For this review, take the finished solid that the model builds, in its own axes (mm). Face numbers are marked on the shaded views. A direction names the side the tool comes from. Round coordinates to 2 decimals unless told otherwise and drop trailing zeros. Order: outer loops, then holes, each group sorted by start corner. A loop starts at its lowest first (then second) coordinate and runs counter-clockwise, first axis right, second up. Notation, with made-up numbers: (54.5, 16.25) -> (97.5, 16.25) arc R18 cw to (97.5, 39.25) -> close; hole circle Ø5 at (-24, 35). An arc over 180 degrees is marked (long way). Use a Markdown table: item, result. Add a question column.
1) Clearance check with flat-ended pins moving along their axes: P1, Ø0.6, axis at x = -73, z = 15.5, coming from the -Y side; P2, Ø16, axis at y = -0.5, z = 84, coming from the +X side; P3, Ø22, axis at y = 9, z = 87.5, coming from the -X side. State where each tip first meets the part, or that it passes through.
2) Consider section C-C (y = -6). State the section outline as (x, z) points, plus the area to 3 significant figures.
3) Consider section A-A (z = 7). Give the number of separate pieces and of enclosed holes in the cut face, plus the area to 3 significant figures.
4) Machinability: for the marked faces 1, 2 and 3, which of the approach directions +Z, -Z, +X, -X, +Y, -Y give a long, thin tool a straight path to every point of the face, cutting with its end or side? Answer none if there is none.
5) Consider section D-D (z = 73.5). State the section outline as (x, y) points.
6) Wall thickness on line 1 along X through (y, z) = (12, 91.5); line 2 along Y through (x, z) = (40.5, 76.2); line 3 along Z through (x, y) = (-33, 0): over which ranges is each line inside the solid? List them lowest first. Write a range as [from, to].
7) Consider section B-B (x = 34.5). State the section outline as (y, z) points, plus the area to 3 significant figures.
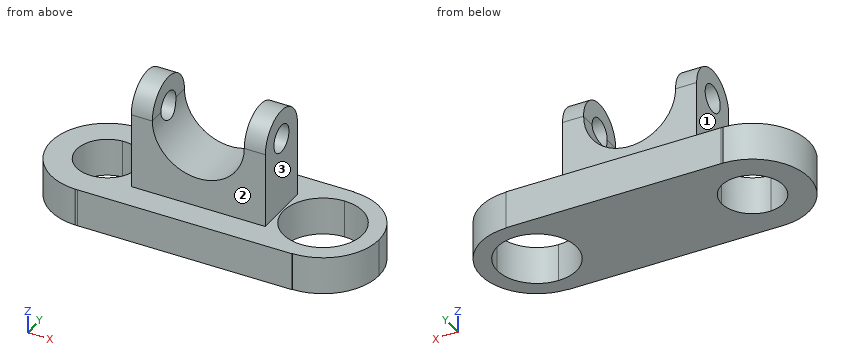
```python
from build123d import *

# Parameters (mm, degrees)
F1_DEPTH  = 76.2
F2_DEPTH  = 25.4
F3_R      = 31.0113659553
F4_DEPTH  = 48.768
F5_W      = 14.2128238031
F5_H      = 19.8651105165
F7_W      = 14.2128238031
F7_H      = 19.8651105165
F9_R      = 9.3175662763
F10_DEPTH = 120.904


with BuildPart() as f1:
    # F0 (on Top) → F1 (new body)
    with BuildSketch(Plane.XY):
        with BuildLine():
            ThreePointArc((-39.4395748653, 19.8651105165), (-35.2913919529, 10.3150682913), (-33.8736140697, 0))
            ThreePointArc((-33.8736140697, 0), (-35.2913919529, -10.3150682913), (-39.4395748653, -19.8651105165))
            Line((-39.4395748653, -19.8651105165), (41.0163370235, -19.8651105165))
            ThreePointArc((41.0163370235, -19.8651105165), (35.3919404434, 0), (41.0163370235, 19.8651105165))
            Line((41.0163370235, 19.8651105165), (-39.4395748653, 19.8651105165))
        make_face()
        with BuildLine():
            ThreePointArc((-39.4395748653, -19.8651105165), (-35.2913919529, -10.3150682913), (-33.8736140697, 0))
            ThreePointArc((-33.8736140697, 0), (-35.2913919529, 10.3150682913), (-39.4395748653, 19.8651105165))
            Line((-39.4395748653, 19.8651105165), (-45.2241897583, 19.8651105165))
            Line((-45.2241897583, 19.8651105165), (-45.2241897583, -19.8651105165))
            Line((-45.2241897583, -19.8651105165), (-39.4395748653, -19.8651105165))
        make_face()
        with BuildLine():
            Line((45.2241897583, 19.8651105165), (41.0163370235, 19.8651105165))
            ThreePointArc((41.0163370235, 19.8651105165), (35.3919404434, 0), (41.0163370235, -19.8651105165))
            Line((41.0163370235, -19.8651105165), (45.2241897583, -19.8651105165))
            Line((45.2241897583, -19.8651105165), (45.2241897583, 19.8651105165))
        make_face()
    extrude(amount=F1_DEPTH)

    # F0 (on Top) → F2 (join)
    with BuildSketch(Plane.XY):
        with BuildLine():
            Line((-45.2241897583, 19.8651105165), (-39.4395748653, 19.8651105165))
            ThreePointArc((-39.4395748653, 19.8651105165), (-53.1034448807, 33.1757028633), (-71.4977306772, 38.2277779281))
            Line((-71.4977306772, 38.2277779281), (-72.7147387814, 38.2277779281))
            ThreePointArc((-72.7147387814, 38.2277779281), (-73.0001282654, 38.2221694419), (-73.2854679227, 38.2144304102))
            Line((-73.2854679227, 38.2144304102), (-73.2854679227, 20.8573796838))
            ThreePointArc((-73.2854679227, 20.8573796838), (-57.7572646523, 15.1831464436), (-51.2155459374, 0))
            ThreePointArc((-51.2155459374, 0), (-57.7572646523, -15.1831464436), (-73.2854679227, -20.8573796838))
            Line((-73.2854679227, -20.8573796838), (-73.2854679227, -38.2144304102))
            ThreePointArc((-73.2854679227, -38.2144304102), (-73.0001282654, -38.2221694419), (-72.7147387814, -38.2277779281))
            Line((-72.7147387814, -38.2277779281), (-71.4977306772, -38.2277779281))
            ThreePointArc((-71.4977306772, -38.2277779281), (-53.1034448807, -33.1757028633), (-39.4395748653, -19.8651105165))
            Line((-39.4395748653, -19.8651105165), (-45.2241897583, -19.8651105165))
            Line((-45.2241897583, -19.8651105165), (-45.2241897583, 19.8651105165))
        make_face()
        with BuildLine():
            ThreePointArc((-71.4977306772, 38.2277779281), (-53.1034448807, 33.1757028633), (-39.4395748653, 19.8651105165))
            Line((-39.4395748653, 19.8651105165), (41.0163370235, 19.8651105165))
            ThreePointArc((41.0163370235, 19.8651105165), (54.80358066, 33.0807990839), (73.2854679227, 37.8935274793))
            Line((73.2854679227, 37.8935274793), (73.2854679227, 38.2277779281))
            Line((73.2854679227, 38.2277779281), (-71.4977306772, 38.2277779281))
        make_face()
        with BuildLine():
            Line((41.0163370235, -19.8651105165), (-39.4395748653, -19.8651105165))
            ThreePointArc((-39.4395748653, -19.8651105165), (-53.1034448807, -33.1757028633), (-71.4977306772, -38.2277779281))
            Line((-71.4977306772, -38.2277779281), (73.2854679227, -38.2277779281))
            Line((73.2854679227, -38.2277779281), (73.2854679227, -37.8935274793))
            ThreePointArc((73.2854679227, -37.8935274793), (54.80358066, -33.0807990839), (41.0163370235, -19.8651105165))
        make_face()
        with BuildLine():
            Line((-72.7147387814, 38.2277779281), (-71.4977306772, 38.2277779281))
            ThreePointArc((-71.4977306772, 38.2277779281), (-72.1062347293, 38.2326206596), (-72.7147387814, 38.2277779281))
        make_face()
        with BuildLine():
            ThreePointArc((73.2854679227, 37.8935274793), (54.80358066, 33.0807990839), (41.0163370235, 19.8651105165))
            Line((41.0163370235, 19.8651105165), (45.2241897583, 19.8651105165))
            Line((45.2241897583, 19.8651105165), (45.2241897583, -19.8651105165))
            Line((45.2241897583, -19.8651105165), (41.0163370235, -19.8651105165))
            ThreePointArc((41.0163370235, -19.8651105165), (54.80358066, -33.0807990839), (73.2854679227, -37.8935274793))
            Line((73.2854679227, -37.8935274793), (73.2854679227, -26.8271780999))
            ThreePointArc((73.2854679227, -26.8271780999), (46.4582898228, 0), (73.2854679227, 26.8271780999))
            Line((73.2854679227, 26.8271780999), (73.2854679227, 37.8935274793))
        make_face()
        with BuildLine():
            ThreePointArc((-72.7147387814, -38.2277779281), (-72.1062347293, -38.2326206596), (-71.4977306772, -38.2277779281))
            Line((-71.4977306772, -38.2277779281), (-72.7147387814, -38.2277779281))
        make_face()
        with BuildLine():
            ThreePointArc((-73.2854679227, 38.2144304102), (-73.0001282654, 38.2221694419), (-72.7147387814, 38.2277779281))
            Line((-72.7147387814, 38.2277779281), (-73.2854679227, 38.2277779281))
            Line((-73.2854679227, 38.2277779281), (-73.2854679227, 38.2144304102))
        make_face()
        with BuildLine():
            ThreePointArc((111.178995402, 0), (100.0802381664, 26.7947702437), (73.2854679227, 37.8935274793))
            Line((73.2854679227, 37.8935274793), (73.2854679227, 26.8271780999))
            ThreePointArc((73.2854679227, 26.8271780999), (92.2551474772, 18.9696795545), (100.1126460226, 0))
            ThreePointArc((100.1126460226, 0), (92.2551474772, -18.9696795545), (73.2854679227, -26.8271780999))
            Line((73.2854679227, -26.8271780999), (73.2854679227, -37.8935274793))
            ThreePointArc((73.2854679227, -37.8935274793), (100.0802381664, -26.7947702437), (111.178995402, 0))
        make_face()
        with BuildLine():
            Line((-73.2854679227, -38.2277779281), (-72.7147387814, -38.2277779281))
            ThreePointArc((-72.7147387814, -38.2277779281), (-73.0001282654, -38.2221694419), (-73.2854679227, -38.2144304102))
            Line((-73.2854679227, -38.2144304102), (-73.2854679227, -38.2277779281))
        make_face()
        with BuildLine():
            Line((-73.2854679227, 20.8573796838), (-73.2854679227, 38.2144304102))
            ThreePointArc((-73.2854679227, 38.2144304102), (-110.3388553889, 0), (-73.2854679227, -38.2144304102))
            Line((-73.2854679227, -38.2144304102), (-73.2854679227, -20.8573796838))
            ThreePointArc((-73.2854679227, -20.8573796838), (-92.9969235211, 0), (-73.2854679227, 20.8573796838))
        make_face()
    extrude(amount=F2_DEPTH)

    # F3 (on face) → F4 (cut)
    with BuildSketch(Plane.XZ.offset(19.8651105165)):
        with Locations((0, 76.2)):
            Circle(F3_R)
    extrude(amount=-F4_DEPTH, mode=Mode.SUBTRACT)

    # F5 (on face) → F6 (revolve)
    with BuildSketch(Plane.XY.offset(76.2)):
        with Locations((-38.1177778568, 9.9325552583)):
            Rectangle(F5_W, F5_H)
    revolve(axis=Axis((-38.1177778568, 0, 76.2), (1, 0, 0)))

    # F7 (on face) → F8 (revolve)
    with BuildSketch(Plane.XY.offset(76.2)):
        with Locations((38.1177778568, 9.9325552583)):
            Rectangle(F7_W, F7_H)
    revolve(axis=Axis((38.1177778568, 0, 76.2), (1, 0, 0)))

    # F9 (on face) → F10 (cut)
    with BuildSketch(Plane.YZ.offset(45.2241897583)):
        with Locations((0, 76.2)):
            Circle(F9_R)
    extrude(amount=-F10_DEPTH, mode=Mode.SUBTRACT)


solid = f1.part
```
Results list:
| question | item | result |
|---|---|---|
| 1 | P1 | y = -38.23 |
| 1 | P2 | x = 45.22 |
| 1 | P3 | x = -45.22 |
| 2 | outline | (-109.87, 0) -> (-92.12, 0) -> (-92.12, 25.4) -> (-109.87, 25.4) -> close; (-52.1, 0) -> (47.14, 0) -> (47.14, 25.4) -> (45.22, 25.4) -> (45.22, 69.07) -> (30.18, 69.07) arc R31.01 cw to (-30.18, 69.07) -> (-45.22, 69.07) -> (-45.22, 25.4) -> (-52.1, 25.4) -> close; (-45.22, 83.33) -> (-31.01, 83.33) -> (-31.01, 95.14) -> (-45.22, 95.14) -> close; (31.01, 83.33) -> (45.22, 83.33) -> (45.22, 95.14) -> (31.01, 95.14) -> close; (99.43, 0) -> (110.7, 0) -> (110.7, 25.4) -> (99.43, 25.4) -> close |
| 2 | area | 6,470 mm2 |
| 3 | separate pieces | 1 |
| 3 | enclosed holes | 2 |
| 3 | area | 12,000 mm2 |
| 4 | face 1 | +Z, -X, +Y, -Y |
| 4 | face 2 | +Z, +X, -X, -Y |
| 4 | face 3 | +Z, +X, +Y, -Y |
| 5 | outline | (-45.22, -19.87) -> (-30.89, -19.87) -> (-30.89, -8.92) -> (-45.22, -8.92) -> close; (-45.22, 8.92) -> (-30.89, 8.92) -> (-30.89, 19.87) -> (-45.22, 19.87) -> close; (30.89, -19.87) -> (45.22, -19.87) -> (45.22, -8.92) -> (30.89, -8.92) -> close; (30.89, 8.92) -> (45.22, 8.92) -> (45.22, 19.87) -> (30.89, 19.87) -> close |
| 6 | line 1 | [-45.22, -31.01], [31.01, 45.22] |
| 6 | line 2 | [-19.87, -9.32], [9.32, 19.87] |
| 6 | line 3 | [0, 66.88], [85.52, 96.07] |
| 7 | outline | (-38.23, 0) -> (38.23, 0) -> (38.23, 25.4) -> (19.87, 25.4) -> (19.87, 76.2) arc R19.87 ccw to (-19.87, 76.2) -> (-19.87, 25.4) -> (-38.23, 25.4) -> close; hole circle Ø18.64 at (0, 76.2) |
| 7 | area | 4,310 mm2 |
